Work out the finished part from the listing and answer in its coordinate system (mm). A direction names the side the tool comes from. Round coordinates to 2 decimals unless told otherwise and drop trailing zeros. Write each loop counter-clockwise with the first axis right and the second up, starting at its lowest first coordinate (ties: lowest second). Pieces come first, ordered by that corner, then holes.
1. Straight lines are drawn through the part: probe 1 along Y at (x, z) = (-0.5, 9.5); probe 2 along Y at (x, z) = (1.25, 1.25); probe 3 along X at (y, z) = (1.05, -1.5). For each, find the intervals that lie inside material, in ascending order.
2. Find section A-A (z = 9). Write down the section's boundary in (x, y), and give its area (3 significant figures).
3. Find section B-B (y = 0.9). Write down the section's boundary in (x, z).
4. Find section C-C (y = -0.2). Write down the section's boundary in (x, z), and give its area (3 significant figures).
5. A tool of negligible diameter and unlimited length cuts with its end or side. For faces 1 (the face through (-2.513, 0.592, 8.409)), 2 (the face through (-2.44, -1.51, 0.54)), 3 (the face through (0, 0, -2)), from which of +Z, -Z, +X, -X, +Y, -Y can it reach the whole face along a straight path? Write none if from no direction.
6. Find section D-D (z = 0). Write down the section's boundary in (x, y), and give its area (3 significant figures).
7. Flat-ended cylindrical pins translate along their axes: pin 1 Ø1.3 at (x, z) = (0.5, -0.5) entering from +Y; pin 2 Ø3.5 at (x, z) = (0.5, 9) entering from -Y. Find the tip coordinate at first contact, or state that the pin passes through.
8. Determine the mould class of faces 4 (the face through (-2, -0.5, 0)), 5 (the face through (-1, 0, 9)), 6 (the face through (-1.978, -1.232, -2.579)) for opening direction X: pulls with the +X half, pulls with the -X half, needs draft (parallel to the pull), parting line crosses it, or undercut.
```python
from build123d import *

# Parameters (mm, degrees)
SKETCH1_R           = 0.5
SKETCH1_R_2         = 3.508270012
SKETCH1_R_3         = 2.25
BOSS_EXTRUDE1_DEPTH = 1.2
SKETCH2_R           = 3.25
SKETCH2_R_2         = 1.5
BOSS_EXTRUDE2_DEPTH = 2.5
SKETCH3_R           = 2.5
CUT_EXTRUDE1_DEPTH  = 2


with BuildPart() as part:
    # Sketch1 → Boss-Extrude1 (new body)
    # profile 1 of 2: a face of its own
    with BuildSketch(Plane(origin=(0, 0, 0), x_dir=(1, 0, 0), z_dir=(0, 1, 0))):
        with BuildLine():
            ThreePointArc((2.882352941, -2), (0, -3.508270012), (-2.882352941, -2))
            Line((-2.882352941, -2), (-2.132352941, -14.999416075))
            ThreePointArc((-2.132352941, -14.999416075), (-0.132626782, -16.99941606), (1.867646984, -14.999963756))
            Line((1.867646984, -14.999963756), (2.882352941, -2))
        make_face()
        with Locations(Location((0, -15, 0), (0, 0, 270))):
            Circle(SKETCH1_R, mode=Mode.SUBTRACT)
        with Locations(Location((0, -13, 0), (0, 0, 270))):
            Circle(SKETCH1_R, mode=Mode.SUBTRACT)
        with Locations(Location((0, -11, 0), (0, 0, 270))):
            Circle(SKETCH1_R, mode=Mode.SUBTRACT)
        with Locations(Location((0, -9, 0), (0, 0, 270))):
            Circle(SKETCH1_R, mode=Mode.SUBTRACT)
        with Locations(Location((0, -7, 0), (0, 0, 270))):
            Circle(SKETCH1_R, mode=Mode.SUBTRACT)
        with Locations(Location((0, -5, 0), (0, 0, 270))):
            Circle(SKETCH1_R, mode=Mode.SUBTRACT)
    # profile 2 of 2: a face of its own
    with BuildSketch(Plane(origin=(0, 0, 0), x_dir=(1, 0, 0), z_dir=(0, 1, 0))):
        Circle(SKETCH1_R_2)
        with Locations(Location((0, 0, 0), (0, 0, 270))):
            Circle(SKETCH1_R_3, mode=Mode.SUBTRACT)
    extrude(amount=BOSS_EXTRUDE1_DEPTH)

    # Sketch2 → Boss-Extrude2 (add)
    with BuildSketch(Plane(origin=(0, 0, 0), x_dir=(1, 0, 0), z_dir=(0, 1, 0))):
        with Locations(Location((0, 0, 0), (0, 0, 270))):
            Circle(SKETCH2_R)
        with Locations(Location((0, 0, 0), (0, 0, 270))):
            Circle(SKETCH2_R_2, mode=Mode.SUBTRACT)
    extrude(amount=-BOSS_EXTRUDE2_DEPTH)

    # Sketch3 → Cut-Extrude1 (cut)
    with BuildSketch(Plane.XZ.offset(2.5)):
        with Locations(Location((0, 0, 0), (0, 0, 270))):
            Circle(SKETCH3_R)
    extrude(amount=-CUT_EXTRUDE1_DEPTH, mode=Mode.SUBTRACT)


solid = part.part
```
Worked answers:
1. probe 1: y = 0 to 1.2
1. probe 2: y = -0.5 to 0
1. probe 3: x = -3.17 to -1.68, 1.68 to 3.17
2. outline: (-2.48, 0) - (-0.5, 0) - (-0.5, 1.2) - (-2.48, 1.2) - close; (0.5, 0) - (2.34, 0) - (2.34, 1.2) - (0.5, 1.2) - close
2. area: 4.58 mm2
3. outline: (-2.88, 2) arc R3.51 ccw (long way) to (2.88, 2) - (1.87, 15) arc R2 ccw to (-2.13, 15) - close; hole circle Ø4.5 at (0, 0); hole circle Ø1 at (0, 5); hole circle Ø1 at (0, 7); hole circle Ø1 at (0, 9); hole circle Ø1 at (0, 11); hole circle Ø1 at (0, 13); hole circle Ø1 at (0, 15)
4. outline: circle Ø6.5 at (0, 0); hole circle Ø3 at (0, 0)
4. area: 26.1 mm2
5. face 1: +Z, -X, +Y, -Y
5. face 2: -Y
5. face 3: +Y
6. outline: (-3.51, 0) - (-3.25, 0) - (-3.25, -2.5) - (-2.5, -2.5) - (-2.5, -0.5) - (-1.5, -0.5) - (-1.5, 0) - (-2.25, 0) - (-2.25, 1.2) - (-3.51, 1.2) - close; (1.5, -0.5) - (2.5, -0.5) - (2.5, -2.5) - (3.25, -2.5) - (3.25, 0) - (3.51, 0) - (3.51, 1.2) - (2.25, 1.2) - (2.25, 0) - (1.5, 0) - close
6. area: 7.77 mm2
7. pin 1: passes through
7. pin 2: stops at y = 0
8. face 4: undercut
8. face 5: needs draft
8. face 6: parting line crosses it
